from build123d import *

# Parameters (mm, degrees)
SKETCH2_W                = 20
SKETCH2_H                = 6
BOSS_EXTRUDE1_DEPTH      = 50
BOSS_EXTRUDE3_DEPTH      = 9
BOSS_EXTRUDE3_DEPTH_BACK = 9
SKETCH6_R                = 2
CUT_EXTRUDE1_DEPTH       = 20
SKETCH7_W                = 20
SKETCH7_H                = 6
BOSS_EXTRUDE4_DEPTH      = 10
FILLET1_R                = 10
FILLET2_R                = 5
FILLET3_R                = 1


with BuildPart() as part:
    # Sketch2 → Boss-Extrude1 (new body)
    with BuildSketch(Plane.XY):
        Rectangle(SKETCH2_W, SKETCH2_H)
    extrude(amount=BOSS_EXTRUDE1_DEPTH)

    # Sketch5 → Boss-Extrude3 (add, two sides: drawn at the far end of the back side and taken through both)
    with BuildSketch(Plane(origin=(0, 0, 0), x_dir=(0, 0, -1), z_dir=(1, 0, 0)).offset(-BOSS_EXTRUDE3_DEPTH_BACK)):
        Polygon((0, -3), (-0.5, -4.8), (-1.25, -4.8), (-1.25, -3), align=None)
    extrude(amount=BOSS_EXTRUDE3_DEPTH + BOSS_EXTRUDE3_DEPTH_BACK)

    # Sketch6 → Cut-Extrude1 (cut)
    with BuildSketch(Plane(origin=(10, 0, 0), x_dir=(0, 0, -1), z_dir=(1, 0, 0))):
        with Locations((-19.5, 0)):
            Circle(SKETCH6_R)
    extrude(amount=-CUT_EXTRUDE1_DEPTH, mode=Mode.SUBTRACT)

    # Sketch7 → Boss-Extrude4 (add)
    with BuildSketch(Plane(origin=(0, 3, 0), x_dir=(1, 0, 0), z_dir=(0, 1, 0))):
        with Locations((0, -47)):
            Rectangle(SKETCH7_W, SKETCH7_H)
    extrude(amount=BOSS_EXTRUDE4_DEPTH)

    # Fillet1
    fillet1_edges = [part.edges().sort_by_distance(p)[0] for p in [
        (0, -3, 50),
    ]]
    fillet(fillet1_edges, radius=FILLET1_R)

    # Fillet2
    fillet2_edges = [part.edges().sort_by_distance(p)[0] for p in [
        (0, 3, 44),
    ]]
    fillet(fillet2_edges, radius=FILLET2_R)

    # Fillet3
    fillet3_edges = [part.edges().sort_by_distance(p)[0] for p in [
        (-10, 13, 47),
        (0, 13, 50),
        (10, 13, 47),
        (0, 13, 44),
    ]]
    fillet(fillet3_edges, radius=FILLET3_R)


solid = part.part
Read the model definition and answer for the solid it produces. Units are mm, in the model's axes. A direction names the side the tool comes from. Round coordinates to 2 decimals unless told otherwise and drop trailing zeros. Order: outer loops, then holes, each group sorted by start corner. A loop starts at its lowest first (then second) coordinate and runs counter-clockwise, first axis right, second up.
1) The mould has two halves that part along Z. Classify faces 1 (the face through (0.1, -1.2, 21.1)), 2 (the face through (0, -4, 1.25)), 3 (the face through (0, 10, 44)), 4 (the face through (10, 1, 25)): released by +Z, released by -Z, zero draft, split by the parting line, or undercut.
2) The part is cut by section B-B on y = 1. Write down the section's boundary in (x, z), plus the area to 3 significant figures.
3) Straight lines are drawn through the part: L1, parallel to Y at x = 3.5, z = 19.5; L2, parallel to Y at x = 3, z = 21; L3, parallel to Y at x = -7.5, z = 10. For each, find the intervals that lie inside material, in ascending order.
4) For faces 5 (the face through (0, 3, 19)), 6 (the face through (9, -4, 1)), 7 (the face through (-9, -4, 1)), 8 (the face through (-9.715, 12.699, 46.958)), determine the directions among +Z, -Z, +X, -X, +Y, -Y from which every point of the face is accessible in a straight line to the end or side of a thin tool.
5) The part is cut by section C-C on x = 1. Write down the section's boundary in (y, z), plus the area to 3 significant figures.
6) Flat-ended cylindrical pins translate along their axes: pin 1 (4.5 mm diameter, centred on x = 0, y = 10.5, fed in from -Z); pin 2 (6 mm diameter, centred on x = 0.5, z = 27, fed in from -Y); pin 3 (5 mm diameter, centred on x = -0.5, z = 11, fed in from +Y). Find the tip coordinate at first contact, or state that the pin passes through.
7) The part is cut by section A-A on z = 19.5. Write down the section's boundary in (x, y), plus the area to 3 significant figures.
8) The part is cut by section D-D on z = 30.5. Write down the section's boundary in (x, y), plus the area to 3 significant figures.
Resolved:
1. face 1: undercut
1. face 2: released by +Z
1. face 3: released by -Z
1. face 4: zero draft
2. outline: (-10, 0) - (10, 0) - (10, 17.77) - (-10, 17.77) - close; (-10, 21.23) - (10, 21.23) - (10, 48) - (-10, 48) - close
2. area: 891 mm2
3. L1: y = -3 to -2, 2 to 3
3. L2: y = -3 to -1.32, 1.32 to 3
3. L3: y = -3 to 3
4. face 5: -Z, +X, -X, +Y
4. face 6: +Z, -Z, +X, -Y
4. face 7: +Z, -Z, -X, -Y
4. face 8: +Z, -Z, -X, +Y
5. outline: (-4.8, 0.5) - (-3, 0) - (3, 0) - (3, 39) arc R5 cw to (8, 44) - (12, 44) arc R1 ccw to (13, 45) - (13, 49) arc R1 ccw to (12, 50) - (7, 50) arc R10 ccw to (-3, 40) - (-3, 1.25) - (-4.8, 1.25) - close; hole circle Ø4 at (0, 19.5)
5. area: 333 mm2
6. pin 1: stops at z = 44
6. pin 2: stops at y = -3
6. pin 3: stops at y = 3
7. outline: (-10, -3) - (10, -3) - (10, -2) - (-10, -2) - close; (-10, 2) - (10, 2) - (10, 3) - (-10, 3) - close
7. area: 40.0 mm2
8. outline: (-10, -3) - (10, -3) - (10, 3) - (-10, 3) - close
8. area: 120 mm2
